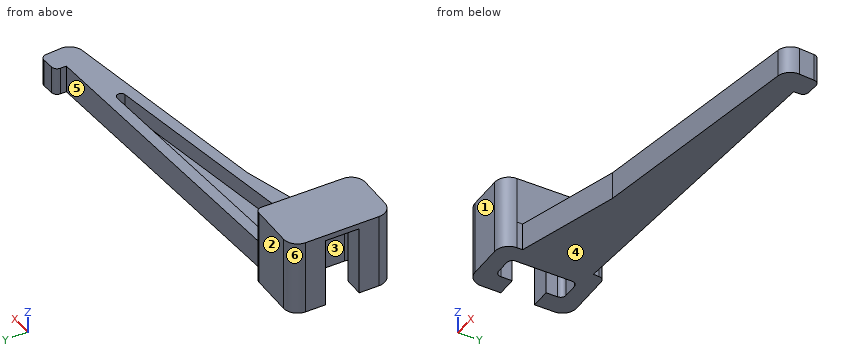
```python
from build123d import *

# Parameters (mm, degrees)
BOSS_EXTRUDE1_DEPTH = 10
BOSS_EXTRUDE2_DEPTH = 10
BOSS_EXTRUDE3_DEPTH = 15
BOSS_EXTRUDE4_DEPTH = 2
CUT_EXTRUDE1_DEPTH  = 6


with BuildPart() as part:
    # Sketch1 → Boss-Extrude1 (new body)
    with BuildSketch(Plane.XY):
        with BuildLine():
            Line((-5, 10), (10.134969828, 10))
            ThreePointArc((10.134969828, 10), (11.498966548, 9.462707403), (12.130097928, 8.139512947))
            Line((12.130097928, 8.139512947), (12.279025895, 6.009743799))
            Line((12.279025895, 6.009743799), (122.011071424, 13.682955911))
            Line((122.011071424, 13.682955911), (122.011071424, 15.827693331))
            ThreePointArc((122.011071424, 15.827693331), (122.54836402, 17.191690051), (123.871558476, 17.822821431))
            Line((123.871558476, 17.822821431), (127.996455725, 18.111262346))
            ThreePointArc((127.996455725, 18.111262346), (129.448086731, 17.625553406), (130.131096773, 16.255647193))
            Line((130.131096773, 16.255647193), (130.513028814, 10.79376454))
            ThreePointArc((130.513028814, 10.79376454), (129.45752894, 7.356802052), (126.3687377, 5.516649939))
            Line((126.3687377, 5.516649939), (12, -14.058605554))
            Line((12, -14.058605554), (12, -21))
            ThreePointArc((12, -21), (10.535533906, -24.535533906), (7, -26))
            Line((7, -26), (-5, -26))
            ThreePointArc((-5, -26), (-8.535533906, -24.535533906), (-10, -21))
            Line((-10, -21), (-10, -14))
            Line((-10, -14), (-3, -14))
            Line((-3, -14), (-3, -18))
            ThreePointArc((-3, -18), (-2.414213562, -19.414213562), (-1, -20))
            Line((-1, -20), (4, -20))
            ThreePointArc((4, -20), (5.414213562, -19.414213562), (6, -18))
            Line((6, -18), (6, 2))
            ThreePointArc((6, 2), (5.414213562, 3.414213562), (4, 4))
            Line((4, 4), (-1, 4))
            ThreePointArc((-1, 4), (-2.414213562, 3.414213562), (-3, 2))
            Line((-3, 2), (-3, -2))
            Line((-3, -2), (-10, -2))
            Line((-10, -2), (-10, 5))
            ThreePointArc((-10, 5), (-8.535533906, 8.535533906), (-5, 10))
        make_face()
    extrude(amount=BOSS_EXTRUDE1_DEPTH)

    # Sketch4 → Boss-Extrude2 (add)
    with BuildSketch(Plane.XY.offset(10)):
        Polygon((12, -18.990256201), (48, -7.896876292), (12, -14.058605554), align=None)
    extrude(amount=-BOSS_EXTRUDE2_DEPTH)

    # Sketch5 → Boss-Extrude3 (add)
    with BuildSketch(Plane.XY.offset(10)):
        with BuildLine():
            Line((12, -21), (12.130097928, 8.139512947))
            ThreePointArc((12.130097928, 8.139512947), (11.498966548, 9.462707403), (10.134969828, 10))
            Line((10.134969828, 10), (-5, 10))
            ThreePointArc((-5, 10), (-8.535533906, 8.535533906), (-10, 5))
            Line((-10, 5), (-10, -2))
            Line((-10, -2), (-3, -2))
            Line((-3, -2), (-3, 2))
            ThreePointArc((-3, 2), (-2.414213562, 3.414213562), (-1, 4))
            Line((-1, 4), (4, 4))
            ThreePointArc((4, 4), (5.414213562, 3.414213562), (6, 2))
            Line((6, 2), (6, -18))
            ThreePointArc((6, -18), (5.414213562, -19.414213562), (4, -20))
            Line((4, -20), (-1, -20))
            ThreePointArc((-1, -20), (-2.414213562, -19.414213562), (-3, -18))
            Line((-3, -18), (-3, -14))
            Line((-3, -14), (-10, -14))
            Line((-10, -14), (-10, -21))
            ThreePointArc((-10, -21), (-8.535533906, -24.535533906), (-5, -26))
            Line((-5, -26), (7, -26))
            ThreePointArc((7, -26), (10.535533906, -24.535533906), (12, -21))
        make_face()
    extrude(amount=BOSS_EXTRUDE3_DEPTH)

    # Sketch6 → Boss-Extrude4 (add)
    with BuildSketch(Plane.XY.offset(25)):
        with BuildLine():
            Line((-10, 5), (-10, -21))
            ThreePointArc((-10, -21), (-8.535533906, -24.535533906), (-5, -26))
            Line((-5, -26), (7, -26))
            ThreePointArc((7, -26), (10.535533906, -24.535533906), (12, -21))
            Line((12, -21), (12.130097928, 8.139512947))
            ThreePointArc((12.130097928, 8.139512947), (11.498966548, 9.462707403), (10.134969828, 10))
            Line((10.134969828, 10), (-5, 10))
            ThreePointArc((-5, 10), (-8.535533906, 8.535533906), (-10, 5))
        make_face()
    extrude(amount=BOSS_EXTRUDE4_DEPTH)

    # Sketch2 → Cut-Extrude1 (cut)
    with BuildSketch(Plane.XY.offset(10)):
        with BuildLine():
            Line((12.07041778, -5.227728761), (12.086053037, -1.725722453))
            ThreePointArc((12.086053037, -1.725722453), (13.166695385, 0.990936179), (15.806987276, 2.246675299))
            Line((15.806987276, 2.246675299), (100.359457674, 8.159159996))
            ThreePointArc((100.359457674, 8.159159996), (101.953365437, 6.84188311), (100.717151126, 5.18431425))
            Line((100.717151126, 5.18431425), (16.745201224, -9.188252997))
            ThreePointArc((16.745201224, -9.188252997), (13.484730649, -8.29754203), (12.07041778, -5.227728761))
        make_face()
    extrude(amount=-CUT_EXTRUDE1_DEPTH, mode=Mode.SUBTRACT)


solid = part.part
```
Here's how the part is built. I have some questions about the finished solid (model axes, mm). Face numbers are marked on the shaded views. A direction names the side the tool comes from. Coordinates: 2 decimals unless noted, no trailing zeros. Loops run counter-clockwise (first coordinate to the right, second up) from the corner with the lowest first, then second, coordinate; pieces in that order, holes last. Notation, with made-up numbers: (29, 86) - (75, 86) arc R21 ccw to (75, 94) - close; hole circle Ø8 at (13, -8.75). An arc over 180 degrees is marked (long way). Answer as CSV lines item,"result".
Q1. If we section it at A-A, the plane z = 19.75: Write out the boundary of the cut face in (x, y), and give its area (3 significant figures).
Response:
outline,"(-10, -21) arc R5 ccw to (-5, -26) - (7, -26) arc R5 ccw to (12, -21) - (12.13, 8.14) arc R2 ccw to (10.13, 10) - (-5, 10) arc R5 ccw to (-10, 5) - (-10, -2) - (-3, -2) - (-3, 2) arc R2 cw to (-1, 4) - (4, 4) arc R2 cw to (6, 2) - (6, -18) arc R2 cw to (4, -20) - (-1, -20) arc R2 cw to (-3, -18) - (-3, -14) - (-10, -14) - close"
area,"481 mm2"
Q2. If we section it at C-C, the plane y = 0.5: Write out the boundary of the cut face in (x, z), and give its area (3 significant figures).
Response:
outline,"(-10, 0) - (-3, 0) - (-3, 25) - (6, 25) - (6, 0) - (97.06, 0) - (97.06, 10) - (73.35, 10) - (73.35, 4) - (12.77, 4) - (12.77, 10) - (12.1, 10) - (12.1, 27) - (-10, 27) - close"
area,"858 mm2"
Q3. If we section it at D-D, the plane x = 78: Write out the boundary of the cut face in (y, z).
Response:
outline,"(-2.76, 0) - (10.61, 0) - (10.61, 10) - (6.6, 10) - (6.6, 4) - (1.3, 4) - (1.3, 10) - (-2.76, 10) - close"
Q4. If we section it at B-B, the plane x = 13.5: Write out the boundary of the cut face in (y, z), and give its area (3 significant figures).
Response:
outline,"(-18.53, 0) - (6.1, 0) - (6.1, 10) - (1.31, 10) - (1.31, 4) - (-8.31, 4) - (-8.31, 10) - (-18.53, 10) - close"
area,"189 mm2"
Q5. If I drill on L1, parallel to X at y = -1, z = 11.75; L2, parallel to X at y = -17, z = 18.75; L3, parallel to Z at x = 44, y = 7, over which ranges is the centre line in solid material (lowest first)? Write a range as [from, to].
Response:
L1,"[-10, -3], [6, 12.09]"
L2,"[-10, -3], [6, 12.02]"
L3,"[0, 10]"
Q6. For pin 1 (2 mm diameter, centred on y = -17, z = 13, fed in from +X); pin 2 (5 mm diameter, centred on x = 62.5, y = 8.5, fed in from +Z); pin 3 (5 mm diameter, centred on x = 10.5, z = 9.5, fed in from +Y); pin 4 (6 mm diameter, centred on y = -12.5, z = 14.5, fed in from -X), each with a flat end and sliding along its axis, tell me the tip position at first contact or that it passes through.
Response:
pin 1,"x = 12.02"
pin 2,"z = 10"
pin 3,"y = 10"
pin 4,"x = -10"
Q7. For the marked faces 1 and 2, which set-ups out of +Z, -Z, +X, -X, +Y, -Y let a thin tool reach every point of the face, with its end or its side?
Response:
face 1,"+Z, -Z, +X, -X, -Y"
face 2,"+Z, -Z, -X, +Y"
Q8. We'd pull the mould along X, two halves only. Please class the marked faces 3, 4, 5 and 6: pulls with the +X half, pulls with the -X half, needs draft (parallel to the pull), parting line crosses it, or undercut.
Response:
face 3,"undercut"
face 4,"needs draft"
face 5,"undercut"
face 6,"pulls with the -X half"
